Could you check a few things on this model? Use its own coordinates, in mm. A direction names the side the tool comes from. Round coordinates to 2 decimals unless told otherwise and drop trailing zeros. Loops run counter-clockwise (first coordinate to the right, second up) from the corner with the lowest first, then second, coordinate; pieces in that order, holes last. Notation, with made-up numbers: M 56.5,49.5 L 74.5,49.5 A21 ccw 74.5,87.5 Z; hole C -1,47 d4. An arc over 180 degrees is marked long. Return JSON: item names as keys, results as strings. Group by question number.
```python
from build123d import *

# Parameters (mm, degrees)
IZIM1_R                     = 20
Y_KSEKLIK_EKSTR_ZYON1_DEPTH = 7
IZIM2_R                     = 10
Y_KSEKLIK_EKSTR_ZYON2_DEPTH = 82
IZIM3_R                     = 3
KES_EKSTR_ZYON1_DEPTH       = 41


with BuildPart() as part:
    # Çizim1 → Yükseklik-Ekstrüzyon1 (new body)
    with BuildSketch(Plane.XY):
        Circle(IZIM1_R)
    extrude(amount=Y_KSEKLIK_EKSTR_ZYON1_DEPTH)

    # Çizim2 → Yükseklik-Ekstrüzyon2 (add)
    with BuildSketch(Plane.XY.offset(7)):
        Circle(IZIM2_R)
    extrude(amount=Y_KSEKLIK_EKSTR_ZYON2_DEPTH)

    # Çizim3 → Kes-Ekstrüzyon1 (cut, symmetric)
    with BuildSketch(Plane(origin=(0, 0, 0), x_dir=(1, 0, 0), z_dir=(0, 1, 0))):
        with Locations(Location((0, -82, 0), (0, 0, 270))):
            Circle(IZIM3_R)
    extrude(amount=KES_EKSTR_ZYON1_DEPTH, both=True, mode=Mode.SUBTRACT)


solid = part.part
```
1. I'm going to push flat-ended pins straight in: pin 1 Ø6 at (y, z) = (-5.5, 66) entering from -X; pin 2 Ø3 at (y, z) = (0, 47) entering from +X; pin 3 Ø12 at (x, z) = (-8.5, 60) entering from -Y. Where does each tip first touch, or does it pass through?
2. I need wall thicknesses on probe 1 along Z at (x, y) = (0, -5.5); probe 2 along X at (y, z) = (0.25, 82); probe 3 along X at (y, z) = (4, 82). Which ranges of each line are inside material? Lowest first, please.
3. We'd pull the mould along X, two halves only. Please class faces 3 (the face through (0, 0, 79)), 4 (the face through (0, 0, 0)), 5 (the face through (9.54, 3, 47.43)): +X half, -X half, draft (parallel to the pull), parting line (faces both ways), or undercut.
4. If we section it at B-B, the plane y = 0: Please give me the cut outline in (x, z), then the cut area to 3 significant figures.
5. If we section it at A-A, the plane x = -1: Please give me the cut outline in (y, z).
6. On a 3-axis mill with a long thin cutter (end or side, diameter ignored), from which of +Z, -Z, +X, -X, +Y, -Y can I reach the whole of each face in a straight line? I mean faces 1 (the face through (-5, 9, 7)), 2 (the face through (-4.336, -19.524, 3.451)). Say none if no direction works.
7. If we section it at C-C, the plane z = 82: Please give me the cut outline in (x, y).
8. If we section it at D-D, the plane x = -7: Please give me the cut outline in (y, z) (3 decimals), then the cut area to 3 significant figures.
Geometry results:
{
 "1": {"pin 1": "x = -9.68", "pin 2": "x = 10", "pin 3": "y = -9.68"},
 "2": {"probe 1": "0 to 79, 85 to 89", "probe 2": "-10 to -3, 3 to 10", "probe 3": "-9.17 to -3, 3 to 9.17"},
 "3": {"face 3": "undercut", "face 4": "draft", "face 5": "parting line"},
 "4": {"outline": "M -20,0 L 20,0 L 20,7 L 10,7 L 10,89 L -10,89 L -10,7 L -20,7 Z; hole C 0,82 d6", "area": "1,890 mm^2"},
 "5": {"outline": "M -19.97,0 L 19.97,0 L 19.97,7 L 9.95,7 L 9.95,79.17 L -9.95,79.17 L -9.95,7 L -19.97,7 Z; M -9.95,84.83 L 9.95,84.83 L 9.95,89 L -9.95,89 Z"},
 "6": {"face 1": "+Z", "face 2": "+Z, -Z"},
 "7": {"outline": "M -3,-9.54 L -3,9.54 A10 ccw Z; M 3,-9.54 A10 ccw 3,9.54 Z"},
 "8": {"outline": "M -18.735,0 L 18.735,0 L 18.735,7 L 7.141,7 L 7.141,89 L -7.141,89 L -7.141,7 L -18.735,7 Z", "area": "1,430 mm^2"}
}
